Check sheet for the modelled part. Datum: model origin and axes. Units: mm. A direction names the side the tool comes from. Coordinates: 2 decimals unless noted, no trailing zeros. Write each loop counter-clockwise with the first axis right and the second up, starting at its lowest first coordinate (ties: lowest second). Pieces come first, ordered by that corner, then holes. Notation, with made-up numbers: (-26.5, 79) - (29.5, 79) arc R24 ccw to (29.5, 106) - close; hole circle Ø8 at (11, -31). An arc over 180 degrees is marked (long way). Use one line per item in the form item = value. Start each with the question number.
1. Cross-section at B-B on x = 171.75. Record the boundary of the cut face in (y, z), then the cut area to 3 significant figures.
2. Go/stop test with flat-tipped pins: pin 1 Ø3.5 at (x, z) = (177.4, -19.5) entering from +Y; pin 2 Ø0.7 at (x, z) = (181.5, -10) entering from -Y. Record where each tip stops, or that it passes through.
3. Scan lines: line 1 along X through (y, z) = (67, -3); line 2 along Z through (x, y) = (178, 63); line 3 along Y through (x, z) = (172, -1.5). Record each from-to range of solid material in increasing order.
4. Draft check along X on faces 4 (the face through (173, 61.559, -11)), 5 (the face through (167.947, 65, -11)), 6 (the face through (177, 62.145, -22)). Enter one of: +X half, -X half, draft (parallel to the pull), parting line (faces both ways), or undercut.
5. Cross-section at A-A on z = -3. Record the boundary of the cut face in (x, y).
6. Tool access check on faces 1 (the face through (181, 62.145, -11)), 2 (the face through (177, 62.145, -11)), 3 (the face through (181.6, 67.9, -11.1)). Record the directions out of +Z, -Z, +X, -X, +Y, -Y that give a thin tool (end or side, any length) a straight path to the whole face; none if there is none.
7. Cross-section at C-C on y = 66.75. Record the boundary of the cut face in (x, z), then the cut area to 3 significant figures.
```python
from build123d import *

# Parameters (mm, degrees)
BOSS_EXTRUDE1_DEPTH = 22.5
SKETCH2_R           = 1.9
CUT_EXTRUDE1_DEPTH  = 184.450850043
FILLET1_R           = 0.5


with BuildPart() as part:
    # Sketch1 → Boss-Extrude1 (new body)
    with BuildSketch(Plane.XY):
        with BuildLine():
            Line((167.946665474, 62.144706948), (167.946665474, 67.144706948))
            ThreePointArc((167.946665474, 67.144706948), (168.239558693, 67.851813729), (168.946665474, 68.144706948))
            Line((168.946665474, 68.144706948), (180.946665474, 68.144706948))
            ThreePointArc((180.946665474, 68.144706948), (181.653772255, 67.851813729), (181.946665474, 67.144706948))
            Line((181.946665474, 67.144706948), (181.946665474, 62.144706948))
            Line((181.946665474, 62.144706948), (180.646665474, 62.144706948))
            Line((180.646665474, 62.144706948), (180.546665474, 61.558713892))
            Line((180.546665474, 61.558713892), (179.746665474, 61.558713892))
            Line((179.746665474, 61.558713892), (179.646665474, 62.144706948))
            Line((179.646665474, 62.144706948), (178.346665474, 62.144706948))
            Line((178.346665474, 62.144706948), (178.246665474, 61.558713892))
            Line((178.246665474, 61.558713892), (177.446665474, 61.558713892))
            Line((177.446665474, 61.558713892), (177.346665474, 62.144706948))
            Line((177.346665474, 62.144706948), (176.046665474, 62.144706948))
            Line((176.046665474, 62.144706948), (175.946665474, 61.558713892))
            Line((175.946665474, 61.558713892), (175.146665474, 61.558713892))
            Line((175.146665474, 61.558713892), (175.046665474, 62.144706948))
            Line((175.046665474, 62.144706948), (173.746665474, 62.144706948))
            Line((173.746665474, 62.144706948), (173.646665474, 61.558713892))
            Line((173.646665474, 61.558713892), (172.846665474, 61.558713892))
            Line((172.846665474, 61.558713892), (172.746665474, 62.144706948))
            Line((172.746665474, 62.144706948), (171.446665474, 62.144706948))
            Line((171.446665474, 62.144706948), (171.346665474, 61.558713892))
            Line((171.346665474, 61.558713892), (170.546665474, 61.558713892))
            Line((170.546665474, 61.558713892), (170.446665474, 62.144706948))
            Line((170.446665474, 62.144706948), (169.146665474, 62.144706948))
            Line((169.146665474, 62.144706948), (169.046665474, 61.558713892))
            Line((169.046665474, 61.558713892), (168.246665474, 61.558713892))
            Line((168.246665474, 61.558713892), (168.146665474, 62.144706948))
            Line((168.146665474, 62.144706948), (167.946665474, 62.144706948))
        make_face()
    extrude(amount=-BOSS_EXTRUDE1_DEPTH)

    # Sketch2 → Cut-Extrude1 (cut, through all)
    with BuildSketch(Plane(origin=(0, 68.144706948, 0), x_dir=(1, 0, 0), z_dir=(0, 1, 0))):
        with Locations(Location((177.403833472, 3, 0), (0, 0, 270))):
            Circle(SKETCH2_R)
        with Locations(Location((177.403833472, 19.5, 0), (0, 0, 270))):
            Circle(SKETCH2_R)
    extrude(amount=-CUT_EXTRUDE1_DEPTH, mode=Mode.SUBTRACT)

    # Fillet1
    fillet1_edges = [part.edges().sort_by_distance(p)[0] for p in [
        (181.946665474, 64.644706948, -22.5),
        (181.653772255, 67.851813729, -22.5),
        (167.946665474, 64.644706948, -22.5),
        (168.239558693, 67.851813729, -22.5),
        (181.946665474, 64.644706948, 0),
        (181.653772255, 67.851813729, 0),
        (167.946665474, 64.644706948, 0),
        (168.239558693, 67.851813729, 0),
        (174.946665474, 68.144706948, -22.5),
        (174.946665474, 68.144706948, 0),
    ]]
    fillet(fillet1_edges, radius=FILLET1_R)


solid = part.part
```
Final values:
q1.outline = (62.14, -22.5) - (67.64, -22.5) arc R0.5 ccw to (68.14, -22) - (68.14, -0.5) arc R0.5 ccw to (67.64, 0) - (62.14, 0) - close
q1.area = 135 mm²
q2.pin_1 = through
q2.pin_2 = 62.14
q3.line_1 = 167.95 to 175.5, 179.3 to 181.95
q3.line_2 = -22.5 to -21.3, -17.7 to -4.8, -1.2 to 0
q3.line_3 = 62.14 to 68.14
q4.face_4 = draft
q4.face_5 = -X half
q4.face_6 = undercut
q5.outline = (167.95, 62.14) - (168.15, 62.14) - (168.25, 61.56) - (169.05, 61.56) - (169.15, 62.14) - (170.45, 62.14) - (170.55, 61.56) - (171.35, 61.56) - (171.45, 62.14) - (172.75, 62.14) - (172.85, 61.56) - (173.65, 61.56) - (173.75, 62.14) - (175.05, 62.14) - (175.15, 61.56) - (175.5, 61.56) - (175.5, 68.14) - (168.95, 68.14) arc R1 ccw to (167.95, 67.14) - close; (179.3, 62.14) - (179.65, 62.14) - (179.75, 61.56) - (180.55, 61.56) - (180.65, 62.14) - (181.95, 62.14) - (181.95, 67.14) arc R1 ccw to (180.95, 68.14) - (179.3, 68.14) - close
q6.face_1 = +Z, -Z, +X, -Y
q6.face_2 = +Z, -Z, -Y
q6.face_3 = +Z, -Z, +X, +Y
q7.outline = (167.95, -22) arc R0.5 ccw to (168.45, -22.5) - (181.45, -22.5) arc R0.5 ccw to (181.95, -22) - (181.95, -0.5) arc R0.5 ccw to (181.45, 0) - (168.45, 0) arc R0.5 ccw to (167.95, -0.5) - close; hole circle Ø3.8 at (177.4, -19.5); hole circle Ø3.8 at (177.4, -3)
q7.area = 292 mm²
